Verification items for the finished model (mm, model axes). Face numbers are marked on the shaded views. Give positions to 0.01 mm unless a question says otherwise; leave off trailing zeros. Order: outer loops, then holes, each group sorted by start corner. A loop starts at its lowest first (then second) coordinate and runs counter-clockwise, first axis right, second up.
(1) Sectioned sample at A-A on x = -5.08. Record the cut outline in (y, z) (1 decimal), plus the area to 3 significant figures.
(2) Sectioned sample at B-B on y = -1.45. Record the cut outline in (x, z), plus the area to 3 significant figures.
(3) Sectioned sample at C-C on z = -24. Record the cut outline in (x, y) (3 decimals), plus the area to 3 significant figures.
(4) Mould release check, pull along Y, two halves, no side actions. Record for the marked faces 1 and 2: pulls with the +Y half, pulls with the -Y half, needs draft (parallel to the pull), parting line crosses it, or undercut.
(5) Scan lines: L1, parallel to Z at x = -5.08, y = -2.45; L2, parallel to Z at x = -5.75, y = -1.5; L3, parallel to X at y = -2.75, z = 26.5. Record each from-to range of solid material in increasing order.
Autodesk Inventor part; units mm, degrees
ref_plane "YZ Plane" through (0, 0, 0) normal (1, 0, 0) x (0, 1, 0)
ref_plane "XZ Plane" through (0, 0, 0) normal (0, 1, 0) x (-1, 0, 0)
ref_plane "XY Plane" through (0, 0, 0) normal (0, 0, 1) x (1, 0, 0)
sketch "Sketch1" plane through (0, 0, 0) normal (0, 1, 0) x (-1, 0, 0)
  line L0 (-2.032, 0) -> (12.192, 0)
  line L1 (0, -40.894) -> (0, 40.894)
  line L2 (10.16, -29.21) -> (0, -29.21)
  line L3 (0, -29.21) -> (0, 29.21)
  line L4 (0, 29.21) -> (10.16, 29.21)
  line L5 (10.16, 29.21) -> (10.16, -29.21)
  line L6 (10.16, -29.21) -> (0, 29.21) construction
  line L7 (0, -29.21) -> (10.16, 29.21) construction
  point P0 (0, 0)
  point P1 (5.08, 0)
  point P2 (5.08, 25.0825)
  point P3 (5.08, 0)
  point P4 (5.08, -25.0825)
  point P5 (0, -29.21)
  dimension "d0" = 58.42
  dimension "d1" = 10.16
  dimension "d2" = 5.08
  dimension "d3" = 25.0825
  dimension "d4" = 25.0825
extrude "Extrusion1" add sketch "Sketch1" against normal blind 3.175
fillet "Fillet1" radius 1.27 2 edges at (-10.16, -1.5875, 29.21) (-10.16, -1.5875, -29.21)
fillet "Fillet2" radius 1.27 2 edges at (0, -1.5875, 29.21) (0, -1.5875, -29.21)
hole "Hole1" at (-5.08, 0, 25.0825) at (-5.08, 0, -25.0825) direction (0, -1, 0) diameter 4.064 end through all
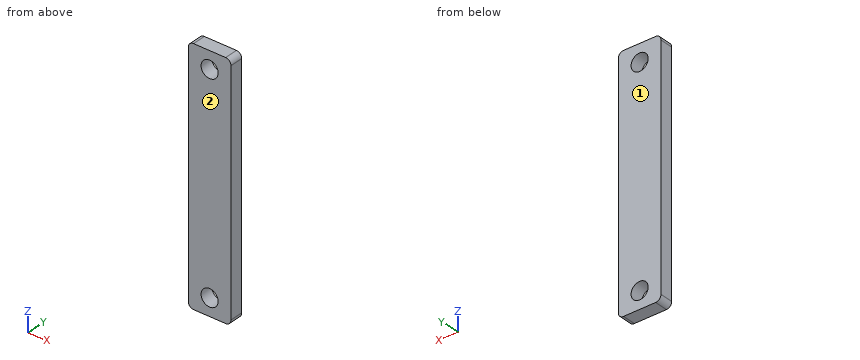
Ans:
1. outline: (-3.2, -29.2) - (0, -29.2) - (0, -27.1) - (-3.2, -27.1) - close; (-3.2, -23.1) - (0, -23.1) - (0, 23.1) - (-3.2, 23.1) - close; (-3.2, 27.1) - (0, 27.1) - (0, 29.2) - (-3.2, 29.2) - close
1. area: 160 mm2
2. outline: (-10.16, -27.94) arc R1.27 ccw to (-8.89, -29.21) - (-1.27, -29.21) arc R1.27 ccw to (0, -27.94) - (0, 27.94) arc R1.27 ccw to (-1.27, 29.21) - (-8.89, 29.21) arc R1.27 ccw to (-10.16, 27.94) - close; hole circle Ø4.06 at (-5.08, -25.08); hole circle Ø4.06 at (-5.08, 25.08)
2. area: 566 mm2
3. outline: (-10.16, -3.175) - (-6.8, -3.175) - (-6.8, 0) - (-10.16, 0) - close; (-3.36, -3.175) - (0, -3.175) - (0, 0) - (-3.36, 0) - close
3. area: 21.3 mm2
4. face 1: pulls with the +Y half
4. face 2: pulls with the -Y half
5. L1: z = -29.21 to -27.11, -23.05 to 23.05, 27.11 to 29.21
5. L2: z = -29.21 to -27, -23.16 to 23.16, 27 to 29.21
5. L3: x = -10.16 to -6.54, -3.62 to 0
